Autodesk Fusion 360 part; units mm, degrees
sketch "Top" plane through (0, 0, 0) normal (0, 0, 1) x (1, 0, 0)
  line L0 (18, 0) -> (138.0004, 0)
  line L1 (148.0004, 10) -> (148.0004, 90)
  line L2 (80.0004, 158) -> (0, 158)
  line L3 (0, 158) -> (0, 58)
  line L4 (18, 0) -> (18, 58)
  line L5 (18, 58) -> (0, 58)
  line L6 (138.0004, 0) -> (148.0004, 10)
  line L7 (80.0004, 158) -> (148.0004, 90)
  line L8 (9, 58) -> (9, 158) construction
  line L9 (18, 49) -> (148.0004, 49) construction
  line L10 (18, 13) -> (148.0004, 13) construction
  line L11 (43, 0) -> (43, 65) construction
  circle A0 centre (9, 79) radius 3.5
  circle A1 centre (9, 139) radius 3.5
  circle A2 centre (43, 49) radius 3.5
  circle A3 centre (118, 49) radius 3.5
  circle A4 centre (43, 13) radius 6
  circle A5 centre (68, 13) radius 3.5
  circle A6 centre (68, 13) radius 7.5
  dimension "d1" = 158
  dimension "d3" = 58
  dimension "d4" = 18
  dimension "d5" = 10
  dimension "d6" = 10
  dimension "d7" = 68
  dimension "d8" = 68
  dimension "d9" = 9
  dimension "d10" = 49
  dimension "d11" = 13
  dimension "d12" = 25
  dimension "d13" = 7
  dimension "d14" = 7
  dimension "d15" = 7
  dimension "d16" = 7
  dimension "d17" = 12
  dimension "d18" = 7
  dimension "d19" = 15
  dimension "d20" = 60
  dimension "d21" = 21
  dimension "d22" = 75
  dimension "d23" = 25
extrude "Extrude1" add sketch "Top" along normal blind 13 contours A6
extrude "Extrude2" add sketch "Top" along normal blind 18 contours L0 L1 L2 L3 L4 L5 L6 L7
sketch "Side" plane through (18, 0, 0) normal (-1, 0, 0) x (0, -1, 0)
  line L0 (-58, 0) -> (0, 0)
  line L1 (0, 0) -> (0, 18)
  line L2 (0, 18) -> (-58, 18)
  line L3 (-58, 18) -> (-58, 0)
  line L4 (0, 0) -> (-58, 0) construction
  line L5 (-58, 0) -> (-58, 18) construction
  line L6 (-58, 18) -> (0, 18) construction
  line L7 (0, 18) -> (0, 0) construction
  line L8 (0, 9) -> (-58, 9) construction
  circle A0 centre (-13, 9) radius 3.5
  dimension "d28" = 7
  dimension "d29" = 13
extrude "Extrude3" cut sketch "Side" against normal blind 35 contours A0
The listing builds one solid part. Answer for the finished solid, in the listing's coordinates (mm). A direction names the side the tool comes from. Coordinates: 2 decimals unless noted, no trailing zeros. Order: outer loops, then holes, each group sorted by start corner. A loop starts at its lowest first (then second) coordinate and runs counter-clockwise, first axis right, second up. Notation, with made-up numbers: (13, 40.25) -> (31, 40.25) arc R10 ccw to (31, 56.25) -> close; hole circle Ø3 at (24, 3.25). An arc over 180 degrees is marked (long way). Answer in a Markdown table with one row per item. Add a question column.
Item 1: Find section B-B (x = 9). Write down the section's boundary in (y, z).
Item 2: Determine the mould class of faces 5 (the face through (114, 124, 9)), 6 (the face through (53, 13, 9)), 7 (the face through (143, 5, 9)), 8 (the face through (73, 80, 0)) for opening direction Y: +Y half, -Y half, draft (parallel to the pull), parting line (faces both ways), or undercut.
Item 3: Which of the six approach directions +Z, -Z, +X, -X, +Y, -Y give full straight-line access (tool end or side, diameter ignored) to faces 1 (the face through (66.2, 9.8, 13)), 2 (the face through (27.923, 13.759, 5.583)), 3 (the face through (73, 80, 18)), 4 (the face through (18, 29, 9))?
Item 4: Find section D-D (z = 15). Write down the section's boundary in (x, y).
Item 5: Find section A-A (y = 13). Write down the section's boundary in (x, z), then the cut area to 3 significant figures.
Item 6: Each of these flat-tipped pins is pushed along its axis until it touches: P1, Ø5, axis at x = 83, z = 10, coming from the +Y side; P2, Ø5.5, axis at y = 13, z = 9, coming from the -X side; P3, Ø3, axis at y = 111, z = 14, coming from the +X side. Where does it stop, or does it pass through?
Item 7: Find the intervals of material crossed by L1, parallel to Y at x = 9, z = 9.5; L2, parallel to Y at x = 49.4, z = 9; L3, parallel to Y at x = 118, z = 10.5, in increasing order. Write a range as from..to.
Item 8: Find section C-C (y = 49). Write down the section's boundary in (x, z).
Result set:
| question | item | result |
|---|---|---|
| 1 | outline | (58, 0) -> (75.5, 0) -> (75.5, 18) -> (58, 18) -> close; (82.5, 0) -> (135.5, 0) -> (135.5, 18) -> (82.5, 18) -> close; (142.5, 0) -> (158, 0) -> (158, 18) -> (142.5, 18) -> close |
| 2 | face 5 | +Y half |
| 2 | face 6 | undercut |
| 2 | face 7 | -Y half |
| 2 | face 8 | draft |
| 3 | face 1 | +Z |
| 3 | face 2 | -X |
| 3 | face 3 | +Z, +X, -X, +Y, -Y |
| 3 | face 4 | +Z, -Z, -X, -Y |
| 4 | outline | (0, 58) -> (18, 58) -> (18, 0) -> (138, 0) -> (148, 10) -> (148, 90) -> (80, 158) -> (0, 158) -> close; hole circle Ø7 at (9, 79); hole circle Ø7 at (9, 139); hole circle Ø12 at (43, 13); hole circle Ø7 at (43, 49); hole circle Ø15 at (68, 13); hole circle Ø7 at (118, 49) |
| 5 | outline | (18, 0) -> (37, 0) -> (37, 5.5) -> (18, 5.5) -> close; (18, 12.5) -> (37, 12.5) -> (37, 18) -> (18, 18) -> close; (49, 0) -> (64.5, 0) -> (64.5, 13) -> (60.5, 13) -> (60.5, 18) -> (49, 18) -> (49, 12.5) -> (53, 12.5) -> (53, 5.5) -> (49, 5.5) -> close; (71.5, 0) -> (148, 0) -> (148, 18) -> (75.5, 18) -> (75.5, 13) -> (71.5, 13) -> close |
| 5 | area | 1,800 mm² |
| 6 | P1 | stops at y = 157.5 |
| 6 | P2 | stops at x = 53 |
| 6 | P3 | stops at x = 128.5 |
| 7 | L1 | y = 58..75.5, 82.5..135.5, 142.5..158 |
| 7 | L2 | y = 0..9.5, 16.5..158 |
| 7 | L3 | y = 0..45.5, 52.5..120 |
| 8 | outline | (18, 0) -> (39.5, 0) -> (39.5, 18) -> (18, 18) -> close; (46.5, 0) -> (114.5, 0) -> (114.5, 18) -> (46.5, 18) -> close; (121.5, 0) -> (148, 0) -> (148, 18) -> (121.5, 18) -> close |
